For this review, use the dimensioned drawing (mm, ordinates from the lowest corner) and the shaded views. A direction names the side the tool comes from. Round coordinates to 2 decimals unless told otherwise and drop trailing zeros. Loops run counter-clockwise (first coordinate to the right, second up) from the corner with the lowest first, then second, coordinate; pieces in that order, holes last. Notation, with made-up numbers: (63.5, 77) - (106.5, 77) arc R21 ccw to (106.5, 106) - close; hole circle Ø11 at (69, 12). An arc over 180 degrees is marked (long way). Use one line per item in the form item = value. Start each with the question number.
(1) We need section B-B, the plane z = 4.1. Write out the cut boundary in (x, y).
(2) Machinability: for the marked faces 1, 2 and 3, which of the approach directions +Z, -Z, +X, -X, +Y, -Y give a long, thin tool a straight path to every point of the face, cutting with its end or side? Answer none if there is none.
(3) Wall thickness on probe 1 along X at (y, z) = (10, 2.45); probe 2 along Y at (x, z) = (29, 1.9); probe 3 along Y at (x, z) = (16.5, 0.65): over which ranges is each line inside the solid? List them lowest first. Write a range as [from, to].
(4) We need section A-A, the plane x = 16. Write out the cut boundary in (y, z), then the cut area to 3 significant figures.
(5) The part is to be moulded in two halves that separate along Y. For the marked faces 4, 5, 6 and 7, say which applies: released by +Y, released by -Y, zero draft, split by the parting line, or undercut.
(6) We need section C-C, the plane y = 6. Write out the cut boundary in (x, z).
(7) We need section D-D, the plane x = 10. Write out the cut boundary in (y, z).
(8) For pin 1 (2 mm diameter, centred on y = 17, z = 0.5, fed in from +X); pin 2 (2.5 mm diameter, centred on x = 27, z = 2.5, fed in from -Y); pin 3 (1 mm diameter, centred on x = 13.5, y = 14, fed in from +Z); pin 4 (2.5 mm diameter, centred on x = 27, z = 1.5, fed in from +Y), all flat-tipped, find the tip position at first contact; note any pin that passes through.
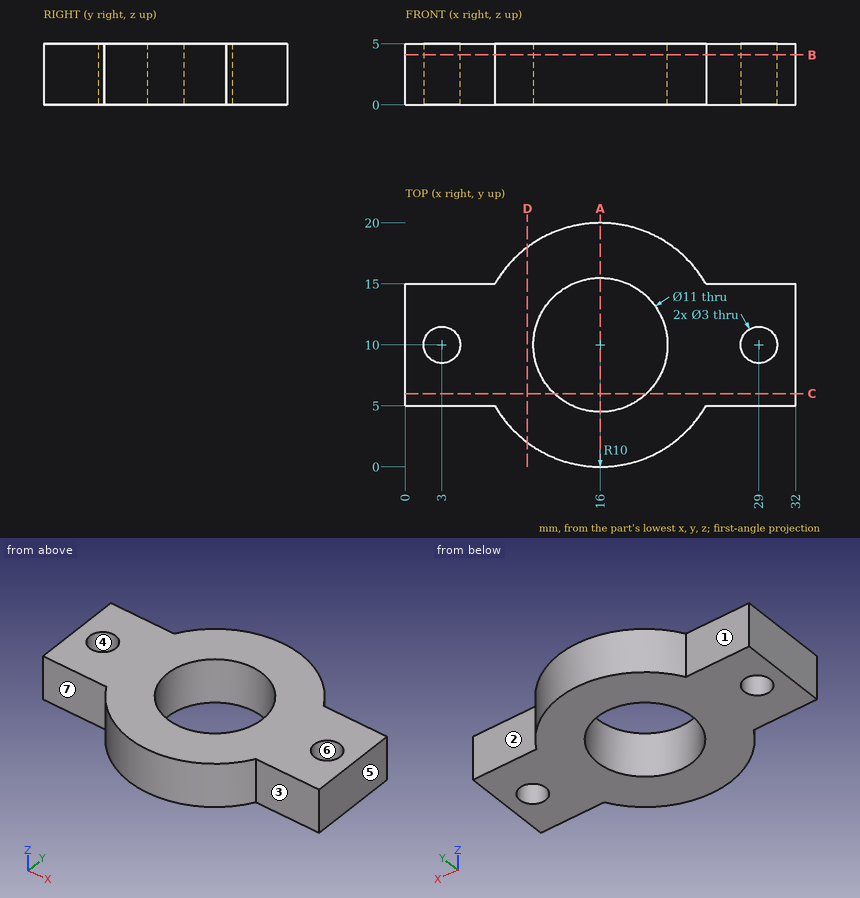
Data:
q1.outline = (0, 5) - (7.34, 5) arc R10 ccw to (24.66, 5) - (32, 5) - (32, 15) - (24.66, 15) arc R10 ccw to (7.34, 15) - (0, 15) - close; hole circle Ø3 at (3, 10); hole circle Ø11 at (16, 10); hole circle Ø3 at (29, 10)
q2.face_1 = +Z, -Z, -X, +Y
q2.face_2 = +Z, -Z, +X, +Y
q2.face_3 = +Z, -Z, +X, -Y
q3.probe_1 = [0, 1.5], [4.5, 10.5], [21.5, 27.5], [30.5, 32]
q3.probe_2 = [5, 8.5], [11.5, 15]
q3.probe_3 = [0.01, 4.52], [15.48, 19.99]
q4.outline = (0, 0) - (4.5, 0) - (4.5, 5) - (0, 5) - close; (15.5, 0) - (20, 0) - (20, 5) - (15.5, 5) - close
q4.area = 45.0 mm^2
q5.face_4 = undercut
q5.face_5 = zero draft
q5.face_6 = undercut
q5.face_7 = released by -Y
q6.outline = (0, 0) - (12.23, 0) - (12.23, 5) - (0, 5) - close; (19.77, 0) - (32, 0) - (32, 5) - (19.77, 5) - close
q7.outline = (2, 0) - (18, 0) - (18, 5) - (2, 5) - close
q8.pin_1 = 24
q8.pin_2 = 5
q8.pin_3 = through
q8.pin_4 = 15
